For this review, use the dimensioned drawing (mm, ordinates from the lowest corner) and the shaded views. A direction names the side the tool comes from. Coordinates: 2 decimals unless noted, no trailing zeros. Loops run counter-clockwise (first coordinate to the right, second up) from the corner with the lowest first, then second, coordinate; pieces in that order, holes last. Notation, with made-up numbers: M -38,70.25 L -17,70.25 A18 ccw -17,94.25 Z; hole C 12.25,71 d11. An arc over 180 degrees is marked long. One line per item, written item: value.
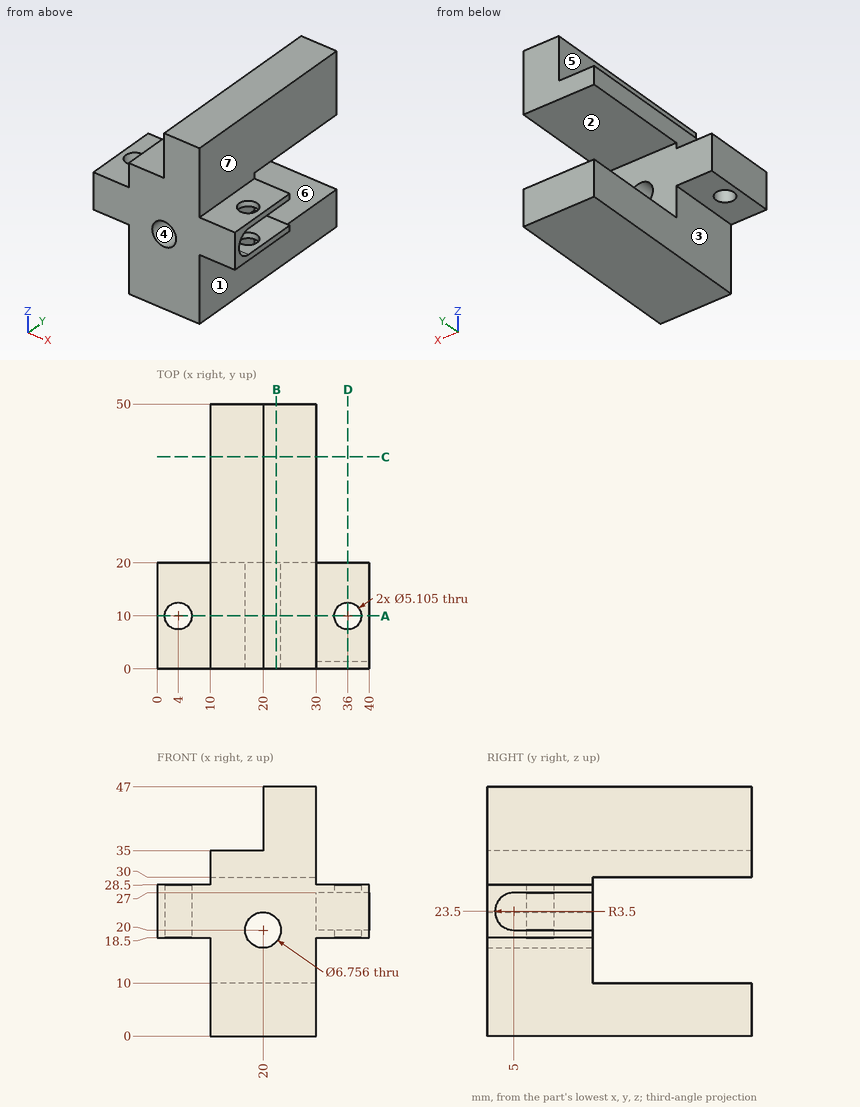
(1) We need section D-D on x = 36. State the section outline as (y, z) points.
Reply:
outline: M 0,18.5 L 7.45,18.5 L 7.45,20 L 5,20 A3.5 cw 5,27 L 7.45,27 L 7.45,28.5 L 0,28.5 Z; M 12.55,18.5 L 20,18.5 L 20,20 L 12.55,20 Z; M 12.55,27 L 20,27 L 20,28.5 L 12.55,28.5 Z
(2) Insertion check: pin 1 (6 mm diameter, centred on x = 27.5, z = 21, fed in from +Y); pin 2 (5 mm diameter, centred on x = 17, y = 24, fed in from +Z); pin 3 (8 mm diameter, centred on x = 5, y = 7, fed in from +Z). Each pin has a flat end and moves straight along its axis. Give the tip position at first contact, or say it passes through.
Reply:
pin 1: stops at y = 20
pin 2: stops at z = 35
pin 3: stops at z = 28.5
(3) We need section A-A on y = 10. State how many separate pieces and enclosed holes the cut face has, then the cut area to 3 significant figures.
Reply:
separate pieces: 4
enclosed holes: 1
area: 848 mm2
(4) Tool access review of the marked faces 5, 6 and 7: name each direction out of +Z, -Z, +X, -X, +Y, -Y from which nothing blocks a thin tool from reaching the whole face with its end or side.
Reply:
face 5: +Z, -X, +Y, -Y
face 6: +X, -X, +Y
face 7: +Z, +X, +Y, -Y
(5) To check wall thickness, follow line 1 along Z through (x, y) = (12.5, 38); line 2 along Z through (x, y) = (29, 30); line 3 along Y through (x, z) = (4, 26.5). State the ranges of each line that lie inside material, in increasing order. Write a range as [from, to].
Reply:
line 1: z = [0, 10], [30, 35]
line 2: z = [0, 10], [30, 47]
line 3: y = [0, 7.45], [12.55, 20]
(6) We need section C-C on y = 40. State the section outline as (x, z) points.
Reply:
outline: M 10,0 L 30,0 L 30,10 L 10,10 Z; M 10,30 L 30,30 L 30,47 L 20,47 L 20,35 L 10,35 Z
(7) Mouldability with a two-part tool opening along X and no side actions: class the marked faces 1, 2, 3 and 4 as released by +X, released by -X, zero draft, split by the parting line, or undercut.
Reply:
face 1: released by +X
face 2: zero draft
face 3: released by -X
face 4: undercut
(8) We need section B-B on x = 22.5. State the section outline as (y, z) points, then the cut area to 3 significant figures.
Reply:
outline: M 0,0 L 50,0 L 50,10 L 20,10 L 20,17.73 L 0,17.73 Z; M 0,22.27 L 20,22.27 L 20,30 L 50,30 L 50,47 L 0,47 Z
area: 1,660 mm2
